```python
from build123d import *

# Parameters (mm, degrees)
SKETCH004_R           = 18
SKETCH004_R_2         = 8
PAD005_DEPTH          = 5
POCKET003_DEPTH       = 3
POLARPATTERN002_COUNT = 4
SKETCH005_R           = 2
PAD006_DEPTH          = 14
POLARPATTERN_COUNT    = 4
SKETCH006_R           = 18
SKETCH006_R_2         = 8
PAD007_DEPTH          = 5
POCKET001_DEPTH       = 5
POLARPATTERN001_COUNT = 4
SKETCH017_R           = 0.8
HOLE_DEPTH            = 9
HOLE_TIPS_R           = 0.8


with BuildPart() as part:
    # Sketch004 → Pad005 (new body)
    with BuildSketch(Plane.XY.offset(3)):
        Circle(SKETCH004_R)
        Circle(SKETCH004_R_2, mode=Mode.SUBTRACT)
    extrude(amount=-PAD005_DEPTH)

    # Sketch016 (on Face4 of Pad005) → Pocket003 (cut)
    with BuildSketch(Plane(origin=(0, 0, -2), x_dir=(1, 0, 0), z_dir=(0, 0, -1))):
        with BuildLine():
            ThreePointArc((-2.274320715, 16.0355366217), (-11.366542794, 11.537446614), (-15.9998121466, 2.5133604465))
            Line((-15.9998121466, 2.5133604465), (-9.3613070154, 1.4705384391))
            ThreePointArc((-1.3306790273, 9.382208997), (-6.6504341316, 6.7504280011), (-9.3613070154, 1.4705384391))
            Line((-2.274320715, 16.0355366217), (-1.3306790273, 9.382208997))
        make_face()
    pocket003 = extrude(amount=-POCKET003_DEPTH, mode=Mode.SUBTRACT)

    # PolarPattern002: Pocket003 ×4 about axis
    polarpattern002_axis = Axis((0, 0, -2), (0, 0, -1))
    for i in range(1, POLARPATTERN002_COUNT):
        add(pocket003.rotate(polarpattern002_axis, i * 360 / POLARPATTERN002_COUNT), mode=Mode.SUBTRACT)

    # Sketch005 (on Face3 of Pad005) → Pad006 (join)
    with BuildSketch(Plane.XY.offset(-2)):
        with Locations((0, 15)):
            Circle(SKETCH005_R)
    pad006 = extrude(amount=-PAD006_DEPTH)

    # PolarPattern: Pad006 ×4 about axis
    polarpattern_axis = Axis((0, 0, 0), (0, 0, 1))
    for i in range(1, POLARPATTERN_COUNT):
        add(pad006.rotate(polarpattern_axis, i * 360 / POLARPATTERN_COUNT))

    # Sketch006 → Pad007 (join)
    with BuildSketch(Plane.XY.offset(-16)):
        Circle(SKETCH006_R)
        Circle(SKETCH006_R_2, mode=Mode.SUBTRACT)
    extrude(amount=-PAD007_DEPTH)

    # Sketch011 (on Face3 of Pad007) → Pocket001 (cut)
    with BuildSketch(Plane(origin=(0, 0, -21), x_dir=(1, 0, 0), z_dir=(0, 0, -1))):
        with BuildLine():
            ThreePointArc((9.2353888952, 1.2979492641), (6.5945841544, 6.5945841544), (1.2979492641, 9.2353888952))
            Line((2.2896869549, 16.2919692324), (1.2979492641, 9.2353888952))
            ThreePointArc((16.2919692324, 2.2896869549), (11.6333771498, 11.6333771498), (2.2896869549, 16.2919692324))
            Line((16.2919692324, 2.2896869549), (9.2353888952, 1.2979492641))
        make_face()
    pocket001 = extrude(amount=-POCKET001_DEPTH, mode=Mode.SUBTRACT)

    # PolarPattern001: Pocket001 ×4 about axis
    polarpattern001_axis = Axis((0, 0, 0), (0, 0, 1))
    for i in range(1, POLARPATTERN001_COUNT):
        add(pocket001.rotate(polarpattern001_axis, i * 360 / POLARPATTERN001_COUNT), mode=Mode.SUBTRACT)

    # Sketch017 (on Face3 of PolarPattern001) → Hole (cut)
    with BuildSketch(Plane(origin=(0, 0, -21), x_dir=(1, 0, 0), z_dir=(0, 0, -1))):
        with Locations((0, 15)):
            Circle(SKETCH017_R)
        with Locations((0, -15)):
            Circle(SKETCH017_R)
        with Locations((-15, 0)):
            Circle(SKETCH017_R)
        with Locations((15, 0)):
            Circle(SKETCH017_R)
    extrude(amount=-HOLE_DEPTH, mode=Mode.SUBTRACT)

    # Hole tips → Hole tip 1 section 0
    with BuildSketch(Plane(origin=(0, 0, -12), x_dir=(1, 0, 0), z_dir=(0, 0, -1)), mode=Mode.PRIVATE) as hole_tip_1_s0:
        with Locations((0, 15)):
            Circle(HOLE_TIPS_R)
    loft([hole_tip_1_s0.sketch, Vertex(0, -15, -11.5193115048)], mode=Mode.SUBTRACT)

    # Hole tips → Hole tip 2 section 0
    with BuildSketch(Plane(origin=(0, 0, -12), x_dir=(1, 0, 0), z_dir=(0, 0, -1)), mode=Mode.PRIVATE) as hole_tip_2_s0:
        with Locations((0, -15)):
            Circle(HOLE_TIPS_R)
    loft([hole_tip_2_s0.sketch, Vertex(0, 15, -11.5193115048)], mode=Mode.SUBTRACT)

    # Hole tips → Hole tip 3 section 0
    with BuildSketch(Plane(origin=(0, 0, -12), x_dir=(1, 0, 0), z_dir=(0, 0, -1)), mode=Mode.PRIVATE) as hole_tip_3_s0:
        with Locations((-15, 0)):
            Circle(HOLE_TIPS_R)
    loft([hole_tip_3_s0.sketch, Vertex(-15, 0, -11.5193115048)], mode=Mode.SUBTRACT)

    # Hole tips → Hole tip 4 section 0
    with BuildSketch(Plane(origin=(0, 0, -12), x_dir=(1, 0, 0), z_dir=(0, 0, -1)), mode=Mode.PRIVATE) as hole_tip_4_s0:
        with Locations((15, 0)):
            Circle(HOLE_TIPS_R)
    loft([hole_tip_4_s0.sketch, Vertex(15, 0, -11.5193115048)], mode=Mode.SUBTRACT)


with BuildPart() as part_1:
    # Body002 placement: moved
    add(part.part.moved(Location((0, 0, -6))))


solid = part_1.part
```
Build history of the part. All positions in model axes, mm. A direction names the side the tool comes from. Round coordinates to 2 decimals unless told otherwise and drop trailing zeros. Write each loop counter-clockwise with the first axis right and the second up, starting at its lowest first coordinate (ties: lowest second). Pieces come first, ordered by that corner, then holes.
1) Band-saw the part on C-C, the plane y = 6. Give the number of separate pieces and of enclosed holes in the cut face, and give its area (3 significant figures).
2) Drill centre lines: probe 1 along Y at (x, z) = (0, -21.5); probe 2 along Y at (x, z) = (-15, -22.5); probe 3 along Y at (x, z) = (-11, -25). Where is each one in solid material? Low to high.
3) Band-saw the part on B-B, the plane z = -7.5. List the corners of the cut face in (x, y), and give its area (3 significant figures).
4) 3-axis set-ups, long thin cutter, end or side, ignore diameter. For faces 1 (the flat face through (7, -5, -22)), 2 (the cylindrical face through (-2.343, 17.847, -24.465)), 3 (the cylindrical face through (6.654, -6.535, -24.535)): which of +Z, -Z, +X, -X, +Y, -Y reach the whole face in a straight line?
5) Band-saw the part on A-A, the plane z = -19.75. List the corners of the cut face in (x, y).
6) Mould opens along Z. For faces 4 (the flat face through (9, -9, -5)), 5 (the flat face through (2, -12.73, -6.52)), 6 (the cylindrical face through (0, -17, -15)) say: +Z half, -Z half, draft (parallel to the pull), parting line (faces both ways), or undercut.
7) Pin check, flat tips, straight feed: pin 1 (6 mm diameter, centred on x = 12, z = -5.5, fed in from +Y); pin 2 (4 mm diameter, centred on x = 12, z = -9.5, fed in from -Y); pin 3 (4.5 mm diameter, centred on x = 9.5, y = 7.5, fed in from -Z). Stop position of each tip, or through.
Ans:
1. separate pieces: 6
1. enclosed holes: 0
1. area: 106 mm2
2. probe 1: y = -17 to -15.8, -14.2 to -13, 13 to 14.2, 15.8 to 17
2. probe 2: y = -9.95 to -6.76, -2.11 to -0.8, 0.8 to 2.11, 6.76 to 9.95
2. probe 3: y = -14.25 to -12.23, -1.55 to 1.55, 12.23 to 14.25
3. outline: circle Ø36 at (0, 0); hole (-16.04, 2.27) - (-9.38, 1.33) arc R9.48 cw to (-1.47, 9.36) - (-2.51, 16) arc R16.2 ccw to start; hole (-16, -2.51) arc R16.2 ccw to (-2.27, -16.04) - (-1.33, -9.38) arc R9.48 cw to (-9.36, -1.47) - close; hole circle Ø16 at (0, 0); hole (1.33, 9.38) arc R9.48 cw to (9.36, 1.47) - (16, 2.51) arc R16.2 ccw to (2.27, 16.04) - close; hole (1.47, -9.36) - (2.51, -16) arc R16.2 ccw to (16.04, -2.27) - (9.38, -1.33) arc R9.48 cw to start
3. area: 377 mm2
4. face 1: none
4. face 2: +Z, -Z
4. face 3: -Z
5. outline: circle Ø4 at (-15, 0); circle Ø4 at (0, -15); circle Ø4 at (0, 15); circle Ø4 at (15, 0); hole circle Ø1.6 at (-15, 0); hole circle Ø1.6 at (0, -15); hole circle Ø1.6 at (0, 15); hole circle Ø1.6 at (15, 0)
6. face 4: -Z half
6. face 5: draft
6. face 6: undercut
7. pin 1: stops at y = 15.59
7. pin 2: stops at y = -14.49
7. pin 3: stops at z = -5
